Here's how the part is built. I have some questions about the finished solid (model axes, mm). A direction names the side the tool comes from. Give positions to 0.01 mm unless a question says otherwise; leave off trailing zeros. Loops run counter-clockwise (first coordinate to the right, second up) from the corner with the lowest first, then second, coordinate; pieces in that order, holes last. Notation, with made-up numbers: (47.25, 78.5) - (82.25, 78.5) arc R16 cw to (82.25, 104.5) - close; hole circle Ø5 at (87, 44). An arc over 180 degrees is marked (long way). Use a Markdown table: item, result.
from build123d import *

# Parameters (mm, degrees)
SKETCH_1_R             = 5.4
EXTRUDE_1_DEPTH        = 39.5
HOLE_WIZARD_M5_2_D     = 4.2
HOLE_WIZARD_M5_2_DEPTH = 12.4
HOLE_WIZARD_M5_2_TIP   = 1.2618073
CHAMFER_2_SIZE         = 0.5
SKETCH_9_R             = 2.75
CUT_EXTRUDE_5_DEPTH    = 2
CHAMFER_3_SIZE         = 0.5
CHAMFER_4_SIZE         = 0.5
HOLE_WIZARD_M5_1_D     = 4.2
HOLE_WIZARD_M5_1_DEPTH = 12.4
HOLE_WIZARD_M5_1_TIP   = 1.2618073
CHAMFER_5_SIZE         = 0.5
SKETCH_11_W            = 10
SKETCH_11_H            = 2
CUT_EXTRUDE_6_DEPTH    = 10


with BuildPart() as part:
    # 草图1 → 拉伸1 (new body)
    with BuildSketch(Plane.XY):
        Circle(SKETCH_1_R)
    extrude(amount=EXTRUDE_1_DEPTH)

    # M5 螺纹孔2
    with Locations(Plane.XY.offset(39.5)):
        with Locations((0, 0)):
            Hole(HOLE_WIZARD_M5_2_D / 2, depth=HOLE_WIZARD_M5_2_DEPTH)
            with Locations((0, 0, -(HOLE_WIZARD_M5_2_DEPTH + HOLE_WIZARD_M5_2_TIP / 2))):  # 118° drill point
                Cone(0, HOLE_WIZARD_M5_2_D / 2, HOLE_WIZARD_M5_2_TIP, mode=Mode.SUBTRACT)

    # 倒角2
    chamfer_2_edges = [part.edges().sort_by_distance(p)[0] for p in [
        (-5.4, 0, 39.5),
    ]]
    chamfer(chamfer_2_edges, length=CHAMFER_2_SIZE)

    # 草图9 → 拉伸5 (cut)
    with BuildSketch(Plane.XY.offset(39.5)):
        Circle(SKETCH_9_R)
    extrude(amount=-CUT_EXTRUDE_5_DEPTH, mode=Mode.SUBTRACT)

    # 倒角3
    chamfer_3_edges = [part.edges().sort_by_distance(p)[0] for p in [
        (-2.75, 0, 39.5),
        (2.1, 0, 37.5),
    ]]
    chamfer(chamfer_3_edges, length=CHAMFER_3_SIZE)

    # 倒角4
    chamfer_4_edges = [part.edges().sort_by_distance(p)[0] for p in [
        (-5.4, 0, 0),
    ]]
    chamfer(chamfer_4_edges, length=CHAMFER_4_SIZE)

    # M5 螺纹孔1
    with Locations(Plane(origin=(0, 0, 0), x_dir=(-1, 0, 0), z_dir=(0, 0, -1))):
        with Locations((0, 0)):
            Hole(HOLE_WIZARD_M5_1_D / 2, depth=HOLE_WIZARD_M5_1_DEPTH)
            with Locations((0, 0, -(HOLE_WIZARD_M5_1_DEPTH + HOLE_WIZARD_M5_1_TIP / 2))):  # 118° drill point
                Cone(0, HOLE_WIZARD_M5_1_D / 2, HOLE_WIZARD_M5_1_TIP, mode=Mode.SUBTRACT)

    # 倒角5
    chamfer_5_edges = [part.edges().sort_by_distance(p)[0] for p in [
        (-2.1, 0, 0),
    ]]
    chamfer(chamfer_5_edges, length=CHAMFER_5_SIZE)

    # 草图11 → 拉伸6 (cut)
    with BuildSketch(Plane.XY):
        with Locations((0, 6)):
            Rectangle(SKETCH_11_W, SKETCH_11_H)
    cut_extrude_6 = extrude(amount=CUT_EXTRUDE_6_DEPTH, mode=Mode.SUBTRACT)

    # 镜向1: 拉伸6 across plane
    add(cut_extrude_6.mirror(Plane.ZX), mode=Mode.SUBTRACT)


solid = part.part
(1) Suppose I cut it at B-B on z = 24. Write out the boundary of the cut face in (x, y), plus the area to 3 significant figures.
A:
| item | result |
|---|---|
| outline | circle Ø10.8 at (0, 0) |
| area | 91.6 mm2 |
(2) Suppose I cut it at A-A on z = 33.5. Write out the boundary of the cut face in (x, y).
A:
| item | result |
|---|---|
| outline | circle Ø10.8 at (0, 0); hole circle Ø4.2 at (0, 0) |
(3) We'd pull the mould along X, two halves only. Please class faces 6 (the face through (0, -5, 5)), 7 (the face through (-0.596, -2.685, 38.26)), 8 (the face through (5.15, 1.62, 19.48)): pulls with the +X half, pulls with the -X half, needs draft (parallel to the pull), parting line crosses it, or undercut.
A:
| item | result |
|---|---|
| face 6 | needs draft |
| face 7 | undercut |
| face 8 | parting line crosses it |
(4) If I drill on line 1 (X direction, y = 0, z = 33.75); line 2 (Y direction, x = 0, z = 38.75), over which ranges is the centre line in solid material (lowest first)?
A:
| item | result |
|---|---|
| line 1 | -5.4 to -2.1, 2.1 to 5.4 |
| line 2 | -5.4 to -2.75, 2.75 to 5.4 |
(5) On a 3-axis mill with a long thin cutter (end or side, diameter ignored), from which of +Z, -Z, +X, -X, +Y, -Y can I reach the whole of each face in a straight line? I mean faces 1 (the face through (-2.003, 0.631, 31.981)), 2 (the face through (2, -2, 0)), 3 (the face through (2.003, 0.631, 6.533)), 4 (the face through (0, 5, 5)), 5 (the face through (-1.2, -3.2, 39.5)). Say none if no direction works.
A:
| item | result |
|---|---|
| face 1 | +Z |
| face 2 | -Z, +X, -X, +Y, -Y |
| face 3 | -Z |
| face 4 | -Z, +X, -X, +Y |
| face 5 | +Z, +X, -X, +Y, -Y |
(6) Will these pins go through, and if not, where does the flat tip stop? pin 1 (2.5 mm diameter, centred on x = 0, y = 0, fed in from -Z); pin 2 (4.5 mm diameter, centred on x = 1, z = 2.5, fed in from +Y); pin 3 (5 mm diameter, centred on y = 3, z = 28.5, fed in from -X).
A:
| item | result |
|---|---|
| pin 1 | z = 12.91 |
| pin 2 | y = 5 |
| pin 3 | x = -5.38 |
